Geometry: final body of the model. Coordinates: model frame, mm. Face numbers are marked on the shaded views. A direction names the side the tool comes from. Round coordinates to 2 decimals unless told otherwise and drop trailing zeros. Loops run counter-clockwise (first coordinate to the right, second up) from the corner with the lowest first, then second, coordinate; pieces in that order, holes last. Notation, with made-up numbers: M -1.75,17 L 24.25,17 A25 ccw 24.25,53 Z; hole C 80.5,34.5 d3. An arc over 180 degrees is marked long. Return JSON: item names as keys, results as strings.
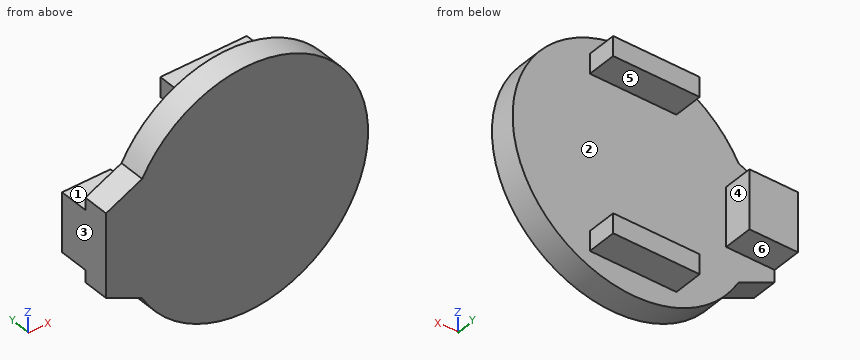
from build123d import *

# Parameters (mm, degrees)
BOSS_EXTRUDE1_DEPTH = 4
SKETCH2_W           = 13.2
SKETCH2_H           = 3
SKETCH2_W_2         = 7.4
SKETCH2_H_2         = 9
BOSS_EXTRUDE2_DEPTH = 4.5


with BuildPart() as part:
    # Sketch1 → Boss-Extrude1 (new body)
    with BuildSketch(Plane(origin=(0, 0, 0), x_dir=(1, 0, 0), z_dir=(0, 1, 0))):
        with BuildLine():
            Line((-21.6, -6.35), (-21.6, 6.35))
            Line((-21.6, 6.35), (-16.079449671, 8.94490348))
            ThreePointArc((-16.079449671, 8.94490348), (18.4, 0), (-16.079449671, -8.94490348))
            Line((-16.079449671, -8.94490348), (-21.6, -6.35))
        make_face()
    extrude(amount=BOSS_EXTRUDE1_DEPTH)

    # Sketch2 → Boss-Extrude2 (add)
    with BuildSketch(Plane(origin=(0, 4, 0), x_dir=(1, 0, 0), z_dir=(0, 1, 0))):
        with Locations((0, 13.285)):
            Rectangle(SKETCH2_W, SKETCH2_H)
        with Locations((0, -13.285)):
            Rectangle(SKETCH2_W, SKETCH2_H)
        with Locations((-17.9, 0)):
            Rectangle(SKETCH2_W_2, SKETCH2_H_2)
    extrude(amount=BOSS_EXTRUDE2_DEPTH)


solid = part.part
Q1. Section query C-C (z = 13). Output: boundary loops of the cut face in (x, y).
Determined:
{"outline": "M -13.02,0 L 13.02,0 L 13.02,4 L 6.6,4 L 6.6,8.5 L -6.6,8.5 L -6.6,4 L -13.02,4 Z"}
Q2. Pull-direction query (Z, two-part tool) for the marked faces 1, 2 and 3; classes: pulls with the +Z half, pulls with the -Z half, needs draft (parallel to the pull), parting line crosses it, or undercut.
Determined:
{"face 1": "pulls with the +Z half", "face 2": "undercut", "face 3": "needs draft"}
Q3. Section query B-B (x = 0). Output: boundary loops of the cut face in (y, z) (3 decimals).
Determined:
{"outline": "M 0,-18.4 L 4,-18.4 L 4,-14.785 L 8.5,-14.785 L 8.5,-11.785 L 4,-11.785 L 4,11.785 L 8.5,11.785 L 8.5,14.785 L 4,14.785 L 4,18.4 L 0,18.4 Z"}
Q4. Material intervals for L1, parallel to Z at x = 2, y = 7.25 (3 decimals); L2, parallel to X at y = 1.75, z = 0.5; L3, parallel to Y at x = 11, z = 10.5, sorted ascending.
Determined:
{"L1": "z = -14.785 to -11.785, 11.785 to 14.785", "L2": "x = -21.6 to 18.39", "L3": "y = 0 to 4"}
Q5. Section query A-A (y = 6). Output: boundary loops of the cut face in (x, z) (3 decimals).
Determined:
{"outline": "M -21.6,-4.5 L -14.2,-4.5 L -14.2,4.5 L -21.6,4.5 Z; M -6.6,-14.785 L 6.6,-14.785 L 6.6,-11.785 L -6.6,-11.785 Z; M -6.6,11.785 L 6.6,11.785 L 6.6,14.785 L -6.6,14.785 Z"}
Q6. Pin query (flat end, axial travel): pin 1 (3.5 mm diameter, centred on y = 6.5, z = 12.5, fed in from -X); pin 2 (5 mm diameter, centred on y = 5.5, z = 0, fed in from +X); pin 3 (0.9 mm diameter, centred on y = 7, z = -13, fed in from +X); pin 4 (1.5 mm diameter, centred on x = 6, y = 3.5, fed in from +Z). Return the tip coordinate at first contact, or that it passes through.
Determined:
{"pin 1": "stops at x = -6.6", "pin 2": "stops at x = 18.4", "pin 3": "stops at x = 6.6", "pin 4": "stops at z = 17.64"}
Q7. Reachability of the marked faces 4, 5 and 6 from +Z, -Z, +X, -X, +Y, -Y: full face, straight path, thin tool, end or side. Return the list, or none.
Determined:
{"face 4": "+Z, -Z, +X, +Y", "face 5": "+X, -X, +Y", "face 6": "-Z, +X, -X, +Y"}
Q8. Section query D-D (y = 0.5). Output: boundary loops of the cut face in (x, z), plus the area to 3 significant figures.
Determined:
{"outline": "M -21.6,-6.35 L -16.08,-8.94 A18.4 ccw long -16.08,8.94 L -21.6,6.35 Z", "area": "1,120 mm^2"}
